Autodesk Inventor part; units mm, degrees
ref_plane "YZ Plane" through (0, 0, 0) normal (1, 0, 0) x (0, 1, 0)
ref_plane "XZ Plane" through (0, 0, 0) normal (0, 1, 0) x (-1, 0, 0)
ref_plane "XY Plane" through (0, 0, 0) normal (0, 0, 1) x (1, 0, 0)
sketch "Sketch1" plane through (0, 0, 0) normal (0, 1, 0) x (-1, 0, 0)
  circle A0 centre (0, 0) radius 14.2875
  line L0 (0, 0) -> (28.7924, 62.2152) construction
  line L1 (0, 0) -> (-39.9389, 3.3748) construction
  line L2 (0, 0) -> (-13.3336, -52.6166) construction
  circle A1 centre (28.7924, 62.2152) radius 3.2512
  circle A2 centre (-39.9389, 3.3748) radius 3.2512
  circle A3 centre (-13.3336, -52.6166) radius 2.54
  line L3 (0, 0) -> (0, 14.2875) construction
  circle A4 centre (28.7924, 62.2152) radius 6.35 construction
  circle A5 centre (-13.3336, -52.6166) radius 6.35 construction
  circle A6 centre (-39.9389, 3.3748) radius 6.35 construction
  circle A7 centre (0, 0) radius 19.05 construction
  line L4 (24.6628, 67.039) -> (-44.0685, 8.1986)
  line L5 (16.8588, -8.8703) -> (-7.714, -55.5734)
  line L6 (18.4713, -4.6596) -> (34.9495, 60.662)
  arc A8 (34.9495, 60.662) -> (24.6628, 67.039) centre (28.7924, 62.2152) ccw
  arc A9 (-44.0685, 8.1986) -> (-45.5031, 0.3151) centre (-39.9389, 3.3748) ccw
  arc A10 (-19.3424, -54.6701) -> (-7.714, -55.5734) centre (-13.3336, -52.6166) ccw
  arc A11 (16.8588, -8.8703) -> (18.4713, -4.6596) centre (0, 0) ccw
  line L7 (-13.3336, -52.6166) -> (-26.0336, -52.6166) construction
  line L8 (-26.0336, -52.6166) -> (-26.0336, -35.0906) construction
  line L9 (-26.0336, -35.0906) -> (-38.7336, -35.0906) construction
  line L10 (-19.3424, -54.6701) -> (-25.9672, -35.285)
  line L11 (-26.1326, -34.9107) -> (-45.5031, 0.3151)
  arc A12 (-25.9672, -35.285) -> (-26.1326, -34.9107) centre (-28.2025, -36.0489) ccw
  dimension "d0" = 28.575
  dimension "d1" = 6.5024
  dimension "d2" = 68.5546
  dimension "d3" = 40.0812
  dimension "d4" = 54.2798
  dimension "d5" = 24.834
  dimension "d8" = 85.17
  dimension "d9" = 12.7
  dimension "d10" = 4.7625
  dimension "d32" = 80.61
  dimension "d33" = 5.08
  dimension "d34" = 12.7
  dimension "d35" = 17.526
  dimension "d36" = 12.7
  dimension "d37" = 2.3622
extrude "Extrusion1" add sketch "Sketch1" along normal blind 4.7625
sketch "Sketch2" plane through (0, 4.7625, 0) normal (0, 1, 0) x (1, 0, 0)
  line L0 (-18.4713, 4.6596) -> (-34.9495, -60.662) construction
  arc A0 (-34.9495, -60.662) -> (-24.6628, -67.039) centre (-28.7924, -62.2152) ccw construction
  line L1 (-24.6628, -67.039) -> (44.0685, -8.1986) construction
  arc A1 (44.0685, -8.1986) -> (45.5031, -0.3151) centre (39.9389, -3.3748) ccw construction
  arc A2 (19.3424, 54.6701) -> (7.714, 55.5734) centre (13.3336, 52.6166) ccw construction
  line L2 (7.714, 55.5734) -> (-16.8588, 8.8703) construction
  arc A3 (-16.8588, 8.8703) -> (-18.4713, 4.6596) centre (0, 0) ccw construction
  circle A4 centre (13.3336, 52.6166) radius 2.54 construction
  circle A5 centre (39.9389, -3.3748) radius 3.2512 construction
  circle A6 centre (-28.7924, -62.2152) radius 3.2512 construction
  circle A7 centre (0, 0) radius 14.2875 construction
  line L3 (-30.3316, -61.8269) -> (-13.8535, 3.4947) construction
  arc A8 (-12.6441, 6.6527) -> (-13.8535, 3.4947) centre (0, 0) ccw construction
  line L4 (-12.6441, 6.6527) -> (11.9287, 53.3558) construction
  arc A9 (14.7675, 53.298) -> (11.9287, 53.3558) centre (13.3336, 52.6166) ccw construction
  line L5 (14.7675, 53.298) -> (41.3727, -2.6935) construction
  arc A10 (40.9713, -4.5808) -> (41.3727, -2.6935) centre (39.9389, -3.3748) ccw construction
  line L6 (40.9713, -4.5808) -> (-27.76, -63.4212) construction
  arc A11 (-30.3316, -61.8269) -> (-27.76, -63.4212) centre (-28.7924, -62.2152) ccw construction
  circle A12 centre (-28.7924, -62.2152) radius 8.0137 construction
  circle A13 centre (0, 0) radius 19.05 construction
  circle A14 centre (39.9389, -3.3748) radius 8.0137 construction
  circle A15 centre (13.3336, 52.6166) radius 7.3025 construction
  line L7 (-25.4267, -54.9426) -> (-8.0008, -17.2884) construction
  line L8 (18.9824, -1.604) -> (31.9536, -2.7001) construction
  line L9 (4.6796, 18.4663) -> (11.5398, 45.5379) construction
  line L10 (-18.5688, -34.4995) -> (-10.9215, -17.975)
  line L11 (-22.7639, -54.8131) -> (-6.6339, -19.9592)
  line L12 (7.4237, 19.6791) -> (13.5496, 43.8526)
  line L13 (2.8441, 20.8396) -> (5.3686, 30.8015)
  line L14 (20.6266, -4.1136) -> (30.5232, -4.9498)
  line L15 (21.0244, 0.5941) -> (30.921, -0.2422)
  arc A16 (-3.9759, -18.6305) -> (18.1565, -5.7656) centre (0, 0) ccw
  arc A17 (-23.1205, -56.554) -> (-22.4788, -57.2797) centre (-28.7924, -62.2152) ccw
  arc A18 (32.5256, -6.4183) -> (33.4711, -8.1063) centre (39.9389, -3.3748) ccw
  line L16 (-19.8865, -56.6807) -> (33.0978, -11.3212)
  arc A19 (-22.7639, -54.8131) -> (-22.4788, -57.2797) centre (-20.6028, -55.8132) ccw
  arc A20 (-23.1205, -56.554) -> (-19.8865, -56.6807) centre (-21.4351, -54.8718) ccw
  arc A21 (-3.9759, -18.6305) -> (-6.6339, -19.9592) centre (-4.4729, -20.9593) ccw
  arc A22 (20.6266, -4.1136) -> (18.1565, -5.7656) centre (20.4261, -6.4864) ccw
  arc A23 (32.5256, -6.4183) -> (30.5232, -4.9498) centre (30.3227, -7.3226) ccw
  arc A24 (33.0978, -11.3212) -> (33.4711, -8.1063) centre (31.5492, -9.5123) ccw
  line L17 (36.9245, 6.668) -> (18.9095, 44.5809)
  arc A25 (18.8666, 2.6372) -> (8.6507, 16.9726) centre (0, 0) ccw
  arc A26 (15.2371, 45.5666) -> (15.9165, 45.7862) centre (13.3336, 52.6166) ccw
  arc A27 (35.9569, 3.5796) -> (33.1414, 0.8694) centre (39.9389, -3.3748) ccw
  arc A28 (7.4237, 19.6791) -> (8.6507, 16.9726) centre (9.732, 19.0941) ccw
  arc A29 (18.8666, 2.6372) -> (21.0244, 0.5941) centre (21.2249, 2.9669) ccw
  arc A30 (30.921, -0.2422) -> (33.1414, 0.8694) centre (31.1215, 2.1306) ccw
  arc A31 (35.9569, 3.5796) -> (36.9245, 6.668) centre (34.7737, 5.646) ccw
  arc A32 (15.2371, 45.5666) -> (13.5496, 43.8526) centre (15.8579, 43.2677) ccw
  arc A33 (18.9095, 44.5809) -> (15.9165, 45.7862) centre (16.7588, 43.5589) ccw
  line L18 (-4.3468, 22.4227) -> (0.9529, 32.4953)
  arc A34 (0.4763, 19.044) -> (-1.9906, 18.9457) centre (0, 0) ccw
  arc A35 (5.3686, 30.8015) -> (0.9529, 32.4953) centre (3.0603, 31.3865) ccw
  arc A36 (-4.3468, 22.4227) -> (-1.9906, 18.9457) centre (-2.2394, 21.3139) ccw
  arc A37 (0.4763, 19.044) -> (2.8441, 20.8396) centre (0.5358, 21.4246) ccw
  line L19 (-23.0388, -32.9169) -> (-18.2122, -13.7837)
  arc A38 (-14.1362, -12.7699) -> (-11.6289, -15.0888) centre (0, 0) ccw
  arc A39 (-23.0388, -32.9169) -> (-18.5688, -34.4995) centre (-20.7298, -33.4994) ccw
  arc A40 (-14.1362, -12.7699) -> (-18.2122, -13.7837) centre (-15.9033, -14.3661) ccw
  arc A41 (-10.9215, -17.975) -> (-11.6289, -15.0888) centre (-13.0825, -16.9749) ccw
  line L20 (45.5031, -0.3151) -> (26.1326, 34.9107)
  arc A42 (25.9672, 35.285) -> (26.1326, 34.9107) centre (28.2025, 36.0489) ccw
  line L21 (25.9672, 35.285) -> (19.3424, 54.6701)
  point P0 (-27.72, -54.2736)
  point P1 (-10.0829, -16.1629)
  point P2 (-23.4325, -56.2578)
  point P3 (-5.7953, -18.1471)
  point P4 (6.9333, 17.7435)
  point P5 (13.926, 45.3382)
  point P6 (2.3536, 18.904)
  point P7 (9.3464, 46.4987)
  point P8 (18.637, -3.9454)
  point P9 (32.1095, -5.0839)
  point P10 (19.0347, 0.7622)
  point P11 (32.5073, -0.3762)
  point P12 (-21.793, -58.3129)
  point P13 (35.0043, -9.689)
  point P14 (38.0016, 4.4012)
  point P15 (17.8266, 46.86)
  point P16 (-6.777, 17.8038)
  point P17 (8.6097, 47.0478)
  point P18 (-28.4103, -54.2106)
  point P19 (-16.9355, -8.7229)
  point P20 (-22.7397, -56.8639)
  dimension "d13" = 4.7625
  dimension "d14" = 4.7625
  dimension "d15" = 4.7625
  dimension "d16" = 4.7625
  dimension "d17" = 4.7625
  dimension "d18" = 2.3622
  dimension "d19" = 2.3622
  dimension "d20" = 2.3622
  dimension "d21" = 2.3622
  dimension "d22" = 2.3622
  dimension "d23" = 2.3622
  dimension "d24" = 2.3813
  dimension "d25" = 2.3813
  dimension "d26" = 2.3813
  dimension "d27" = 2.3813
  dimension "d28" = 2.3813
  dimension "d29" = 2.3813
extrude "Extrusion2" cut sketch "Sketch2" against normal blind 4.7625 contours A39 L19 A40 A38 A41 L10 | L11 A21 A16 A22 L14 A23 A18 A24 L16 A20 A19 | L12 A32 A26 A33 L17 A31 A27 A30 L15 A29 A25 A28 | A37 A34 A36 L18 A35 L13
properties part number "ELEV_036_SPRKTBRKT1" material "Aluminum 6061"
Could you check a few things on this model? Use its own coordinates, in mm. A direction names the side the tool comes from. Round coordinates to 2 decimals unless told otherwise and drop trailing zeros. Write each loop counter-clockwise with the first axis right and the second up, starting at its lowest first coordinate (ties: lowest second). Pieces come first, ordered by that corner, then holes.
(1) If I drill on probe 1 along Z at (x, y) = (2, 3.8); probe 2 along X at (y, z) = (0.55, 10); probe 3 along Z at (x, y) = (-8.5, 2.5), over which ranges is the centre line in solid material (lowest first)?
Findings below:
probe 1: z = -44.71 to -33.52, -19.55 to -14.15, 14.15 to 18.94, 37.94 to 44.21
probe 2: x = -22.17 to -10.2, 10.2 to 16.21, 33.88 to 41.96
probe 3: z = -24.76 to -11.48, 11.48 to 23.99, 46.93 to 53.2
(2) Thinking about a two-plate mould opening in X: for faces 1 (the face through (-20.66, 2.41, 23.48)), 2 (the face through (14.274, 2.348, -0.628)), 3 (the face through (35.682, 2.348, -17.544)), 4 (the face through (-3, 4.762, 15)), which applies, +X half, -X half, draft (parallel to the pull), parting line (faces both ways), or undercut?
Findings below:
face 1: undercut
face 2: undercut
face 3: +X half
face 4: draft
(3) For pin 1 (1 mm diameter, centred on y = 2, z = -44, fed in from +X); pin 2 (1 mm diameter, centred on y = 1, z = 36, fed in from -X), each with a flat end and sliding along its axis, tell me the tip position at first contact or that it passes through.
Findings below:
pin 1: stops at x = 23.16
pin 2: stops at x = -28.85
(4) Suppose I cut it at B-B on x = -29.5. Write out the boundary of the cut face in (y, z), and give its area (3 significant figures).
Findings below:
outline: (0, 39.06) - (4.76, 39.06) - (4.76, 59.04) - (0, 59.04) - close; (0, 65.39) - (4.76, 65.39) - (4.76, 68.53) - (0, 68.53) - close
area: 110 mm2
(5) Suppose I cut it at C-C on y = 2.5. State how many separate pieces and enclosed holes the cut face has, and give its area (3 significant figures).
Findings below:
separate pieces: 1
enclosed holes: 8
area: 2,360 mm2
(6) Suppose I cut it at A-A on z = 53. Write out the boundary of the cut face in (x, y), and give its area (3 significant figures).
Findings below:
outline: (-33.02, 0) - (-21.92, 0) - (-21.92, 4.76) - (-33.02, 4.76) - close; (-15.59, 0) - (-8.26, 0) - (-8.26, 4.76) - (-15.59, 4.76) - close
area: 87.7 mm2
(7) Which directions (+Z, -Z, +X, -X, +Y, -Y) give clear straight access to the entire face, cutting with the end or side of a thin tool? Please do faces 5 (the face through (9.22, 2.35, 38.03)), 6 (the face through (-14.799, 2.415, 26.353)).
Findings below:
face 5: +Z, +X, +Y, -Y
face 6: +Y, -Y
